```python
from build123d import *

# Parameters (mm, degrees)
F1_DEPTH = 0.75
F2_DEPTH = 1
F4_DEPTH = 0.75
F6_DEPTH = 0.75
F8_DEPTH = 0.75


with BuildPart() as f1:
    # F0 (on Top) → F1 (new body)
    with BuildSketch(Plane.XY):
        with BuildLine():
            add(Edge.make_bspline(
                [(-37.5, 18.7313321615), (-32.3807911431, 17.926577975), (-18.7011737223, 16.5680764405), (-7.3513992733, 15.9357535011), (0, 15.7313321615)],
                knots=[0, 0, 0, 0, 0.4901565124, 1, 1, 1, 1], degree=3))
            Line((-37.5, 18.7313321615), (-47, -23.1548529118))
            Line((-47, -23.1548529118), (-16.0084403101, -23.1548529118))
            Line((-16.0084403101, -23.1548529118), (-16.0063231241, -23.0646254072))
            add(Edge.make_bspline(
                [(-43.315390494, -20.4723017862), (-38.3905339247, -21.2993483436), (-33.0056838871, -22.2189238519), (-21.2861009313, -22.8925835376), (-16.0063231241, -23.0646254072)],
                knots=[0, 0, 0, 0, 0.398937465, 0.6969379575, 0.6969379575, 0.6969379575, 0.6969379575], degree=3))
            Line((-43.315390494, -20.4723017862), (-42.7131794367, -17.8171098074))
            Line((-42.7131794367, -17.8171098074), (-43.4446029246, -17.651219237))
            Line((-43.4446029246, -17.651219237), (-36.3666052528, 13.5561829132))
            Line((-36.3666052528, 13.5561829132), (-35.635181765, 13.3902923427))
            Line((-35.635181765, 13.3902923427), (-35.1425150574, 15.562495384))
            add(Edge.make_bspline(
                [(-35.1425150574, 15.562495384), (-30.4836686701, 14.6303577349), (-22.7091897663, 13.9291012054), (-15.9390947662, 13.4553124867), (-14.8013141006, 13.3810050341)],
                knots=[0, 0, 0, 0, 0.4908367268, 0.5909725979, 0.5909725979, 0.5909725979, 0.5909725979], degree=3))
            Line((-14.8013141006, 13.3810050341), (-14.8013141006, 14.1310050341))
            Line((-14.8013141006, 14.1310050341), (-8.8108518429, 13.792830613))
            Line((-8.8108518429, 13.792830613), (-8.8108518429, 13.042830613))
            add(Edge.make_bspline(
                [(-8.8108518429, 13.042830613), (-6.0913133604, 12.9141276056), (-3.2370188614, 12.8126642043), (0, 12.7313321615)],
                knots=[0.7661743328, 0.7661743328, 0.7661743328, 0.7661743328, 1, 1, 1, 1], degree=3))
            Line((0, 12.7313321615), (0, 15.7313321615))
        make_face()
        with BuildLine():
            Line((-16.0084403101, -23.1548529118), (-47, -23.1548529118))
            add(Edge.make_bspline(
                [(-47, -23.1548529118), (-39.471310208, -24.0545421828), (-29.2503257197, -25.7571688291), (-8.0323131497, -26.1634826516), (0, -26.1548529118)],
                knots=[0, 0, 0, 0, 0.4528935937, 1, 1, 1, 1], degree=3))
            Line((0, -26.1548529118), (0, -23.1548529118))
            add(Edge.make_bspline(
                [(-10.0079742572, -23.2053765011), (-6.5667353079, -23.2536816802), (-3.1521121944, -23.2431206783), (0, -23.1548529118)],
                knots=[0.8085428965, 0.8085428965, 0.8085428965, 0.8085428965, 1, 1, 1, 1], degree=3))
            Line((-10.0079742572, -23.2053765011), (-10.0255681439, -23.9551701095))
            Line((-10.0255681439, -23.9551701095), (-16.0239170108, -23.8144190156))
            Line((-16.0239170108, -23.8144190156), (-16.0084403101, -23.1548529118))
        make_face()
        with BuildLine():
            Line((-16.0063231241, -23.0646254072), (-16.0084403101, -23.1548529118))
            Line((-16.0084403101, -23.1548529118), (-12.748052928, -23.1548529118))
            add(Edge.make_bspline(
                [(-16.0063231241, -23.0646254072), (-14.9289009553, -23.0997332718), (-13.8402912127, -23.1300103495), (-12.748052928, -23.1548529118)],
                knots=[0.6969379575, 0.6969379575, 0.6969379575, 0.6969379575, 0.7577496714, 0.7577496714, 0.7577496714, 0.7577496714], degree=3))
        make_face()
        with BuildLine():
            Line((-12.748052928, -23.1548529118), (-16.0084403101, -23.1548529118))
            Line((-16.0084403101, -23.1548529118), (-16.0239170108, -23.8144190156))
            Line((-16.0239170108, -23.8144190156), (-10.0255681439, -23.9551701095))
            Line((-10.0255681439, -23.9551701095), (-10.0079742572, -23.2053765011))
            add(Edge.make_bspline(
                [(-12.748052928, -23.1548529118), (-11.8357565687, -23.1756027605), (-10.9209287599, -23.192561224), (-10.0079742572, -23.2053765011)],
                knots=[0.7577496714, 0.7577496714, 0.7577496714, 0.7577496714, 0.8085428965, 0.8085428965, 0.8085428965, 0.8085428965], degree=3))
        make_face()
        with BuildLine():
            add(Edge.make_bspline(
                [(-14.8013141006, 13.3810050341), (-12.8106074305, 13.2509937357), (-10.8485573953, 13.1392656642), (-8.8108518429, 13.042830613)],
                knots=[0.5909725979, 0.5909725979, 0.5909725979, 0.5909725979, 0.7661743328, 0.7661743328, 0.7661743328, 0.7661743328], degree=3))
            Line((-8.8108518429, 13.042830613), (-8.8108518429, 13.792830613))
            Line((-8.8108518429, 13.792830613), (-14.8013141006, 14.1310050341))
            Line((-14.8013141006, 14.1310050341), (-14.8013141006, 13.3810050341))
        make_face()
        Polygon((-43.4446029246, -17.651219237), (-42.7131794367, -17.8171098074), (-35.635181765, 13.3902923427), (-36.3666052528, 13.5561829132), align=None)
    extrude(amount=F1_DEPTH)

    # F0 (on Top) → F2 (join)
    with BuildSketch(Plane.XY):
        with BuildLine():
            Line((-16.0063231241, -23.0646254072), (-16.0084403101, -23.1548529118))
            Line((-16.0084403101, -23.1548529118), (-12.748052928, -23.1548529118))
            add(Edge.make_bspline(
                [(-16.0063231241, -23.0646254072), (-14.9289009553, -23.0997332718), (-13.8402912127, -23.1300103495), (-12.748052928, -23.1548529118)],
                knots=[0.6969379575, 0.6969379575, 0.6969379575, 0.6969379575, 0.7577496714, 0.7577496714, 0.7577496714, 0.7577496714], degree=3))
        make_face()
        with BuildLine():
            Line((-12.748052928, -23.1548529118), (-16.0084403101, -23.1548529118))
            Line((-16.0084403101, -23.1548529118), (-16.0239170108, -23.8144190156))
            Line((-16.0239170108, -23.8144190156), (-10.0255681439, -23.9551701095))
            Line((-10.0255681439, -23.9551701095), (-10.0079742572, -23.2053765011))
            add(Edge.make_bspline(
                [(-12.748052928, -23.1548529118), (-11.8357565687, -23.1756027605), (-10.9209287599, -23.192561224), (-10.0079742572, -23.2053765011)],
                knots=[0.7577496714, 0.7577496714, 0.7577496714, 0.7577496714, 0.8085428965, 0.8085428965, 0.8085428965, 0.8085428965], degree=3))
        make_face()
        with BuildLine():
            add(Edge.make_bspline(
                [(-14.8013141006, 13.3810050341), (-12.8106074305, 13.2509937357), (-10.8485573953, 13.1392656642), (-8.8108518429, 13.042830613)],
                knots=[0.5909725979, 0.5909725979, 0.5909725979, 0.5909725979, 0.7661743328, 0.7661743328, 0.7661743328, 0.7661743328], degree=3))
            Line((-8.8108518429, 13.042830613), (-8.8108518429, 13.792830613))
            Line((-8.8108518429, 13.792830613), (-14.8013141006, 14.1310050341))
            Line((-14.8013141006, 14.1310050341), (-14.8013141006, 13.3810050341))
        make_face()
        Polygon((-43.4446029246, -17.651219237), (-42.7131794367, -17.8171098074), (-35.635181765, 13.3902923427), (-36.3666052528, 13.5561829132), align=None)
    extrude(amount=-F2_DEPTH)

    # F3 (on face) → F4 (join, through all)
    with BuildSketch(Plane.XY.offset(0.75)):
        Polygon((-47.9752313172, -22.9336654846), (-47, -23.1548529118), (-37.5, 18.7313321615), (-38.4752313172, 18.9525195888), align=None)
    extrude(amount=-F4_DEPTH)

    # F5 (on face) → F6 (join, through all)
    with BuildSketch(Plane.XY.offset(0.75)):
        with BuildLine():
            Line((-38.1434501763, 20.4153665646), (-38.4752313172, 18.9525195888))
            Line((-38.4752313172, 18.9525195888), (-37.5, 18.7313321615))
            add(Edge.make_bspline(
                [(-37.5, 18.7313321615), (-32.3807911431, 17.926577975), (-18.7011737223, 16.5680764405), (-7.3513992733, 15.9357535011), (0, 15.7313321615)],
                knots=[0, 0, 0, 0, 0.4901565124, 1, 1, 1, 1], degree=3))
            Line((0, 15.7313321615), (0, 17.2313321615))
            Line((0, 17.2313321615), (-3.3217752352, 17.2313321615))
            Line((-3.3217752352, 17.2313321615), (-18.8273077893, 18.2105369309))
            Line((-18.8273077893, 18.2105369309), (-38.1434501763, 20.4153665646))
        make_face()
    extrude(amount=-F6_DEPTH)

    # F7 (on face) → F8 (join, through all)
    with BuildSketch(Plane.XY.offset(0.75)):
        with BuildLine():
            Line((-47, -23.1548529118), (-47.9752313172, -22.9336654846))
            Line((-47.9752313172, -22.9336654846), (-48.6002014355, -25.6892038047))
            Line((-48.6002014355, -25.6892038047), (-31.8084545434, -28.2887462527))
            Line((-31.8084545434, -28.2887462527), (-11.6026224568, -29.4112917036))
            Line((-11.6026224568, -29.4112917036), (0, -29.9293901771))
            Line((0, -29.9293901771), (0, -26.1548529118))
            add(Edge.make_bspline(
                [(-47, -23.1548529118), (-39.471310208, -24.0545421828), (-29.2503257197, -25.7571688291), (-8.0323131497, -26.1634826516), (0, -26.1548529118)],
                knots=[0, 0, 0, 0, 0.4528935937, 1, 1, 1, 1], degree=3))
        make_face()
    extrude(amount=-F8_DEPTH)

    # F9 (on face) → F11 section 0
    with BuildSketch(Plane.YZ.offset(-8.8108518429)):
        Polygon((13.792830613, -0.5), (13.792830613, -1), (15.6468802348, -1.75), (15.6468802348, -1.25), align=None)
    # F10 (on face) → F11 section 1
    with BuildSketch(Plane(origin=(-14.8013141006, 0, 0), x_dir=(0, -1, 0), z_dir=(-1, 0, 0))):
        Polygon((-15.9850546559, -1.75), (-14.1310050341, -1), (-14.1310050341, -0.5), (-15.9850546559, -1.25), align=None)
    loft()

    # F12 (on face) → F14 section 0
    with BuildSketch(Plane(origin=(-15.4566018313, 0.3626887438, 0), x_dir=(-0.0234585156, -0.9997248112, 0), z_dir=(-0.9997248112, 0.0234585156, 0))):
        Polygon((24.1837628611, -0.5), (24.1837628611, -1), (26.0378124829, -1.75), (26.0378124829, -1.25), align=None)
    # F13 (on face) → F14 section 1
    with BuildSketch(Plane(origin=(-9.4582529644, 0.2219376499, 0), x_dir=(0.0234585156, 0.9997248112, 0), z_dir=(0.9997248112, -0.0234585156, 0))):
        Polygon((-26.0378124829, -1.75), (-24.1837628611, -1), (-24.1837628611, -0.5), (-26.0378124829, -1.25), align=None)
    loft()

    # F15 (on face) → F17 section 0
    with BuildSketch(Plane(origin=(1.1449940284, 5.04836124, 0), x_dir=(-0.9752313172, 0.2211874272, 0), z_dir=(0.2211874272, 0.9752313172, 0))):
        Polygon((38.4643095643, -0.5), (38.4643095643, -1), (40.3183591861, -1.75), (40.3183591861, -1.25), align=None)
    # F16 (on face) → F17 section 1
    with BuildSketch(Plane(origin=(-5.9330036433, -26.1590409101, 0), x_dir=(0.9752313172, -0.2211874272, 0), z_dir=(-0.2211874272, -0.9752313172, 0))):
        Polygon((-40.3183591861, -1.75), (-38.4643095643, -1), (-38.4643095643, -0.5), (-40.3183591861, -1.25), align=None)
    loft()

    # F18: F1 across plane


with BuildPart() as f1_1:
    add(f1.part)
    add(f1.part.mirror(Plane.YZ))


solid = f1_1.part
```
Check sheet for the modelled part. Datum: model origin and axes. Units: mm. A direction names the side the tool comes from. Give positions to 0.01 mm unless a question says otherwise; leave off trailing zeros. Return JSON: item names as keys, results as strings.
1. Mould release check, pull along X, two halves, no side actions. Record for faces 5 (the flat face through (28.35, 19.298, 0.38)), 6 (the flat face through (43.609, -17.614, -0.856)), 7 (the flat face through (-3, -25, 0.75)), 8 (the flat face through (-40.32, -26.97, 0.38)): +X half, -X half, draft (parallel to the pull), parting line (faces both ways), or undercut.
From the geometry:
{"face 5": "undercut", "face 6": "+X half", "face 7": "draft", "face 8": "-X half"}
2. Material ranges on probe 1 along X at (y, z) = (-16.5, -0.2); probe 2 along X at (y, z) = (-12, 0.65); probe 3 along Y at (x, z) = (4, 0.2), recorded low to high. Write a range as [from, to].
From the geometry:
{"probe 1": "[-43.18, -42.41], [42.41, 43.18]", "probe 2": "[-45.5, -41.39], [41.39, 45.5]", "probe 3": "[-29.75, -23.23], [12.85, 17.27]"}
3. Set-up check for faces 1 (the flat face through (-43.609, -17.614, -0.856)), 2 (the flat face through (-39.856, -1.829, -0.246)), 3 (the flat face through (39.6, -2.1, -1)), 4 (the flat face through (39.856, -1.829, -0.246)): record each of +Z, -Z, +X, -X, +Y, -Y from which the full face is reachable in a straight line by a thin tool's end or side.
From the geometry:
{"face 1": "-Z, -X, -Y", "face 2": "-X, +Y", "face 3": "-Z, -Y", "face 4": "+X, +Y"}
4. Go/stop test with flat-tipped pins: P1, Ø6, axis at x = -39, y = -5, coming from the -Z side; P2, Ø4, axis at x = 38, y = 5, coming from the -Z side; P3, Ø1.2, axis at x = -11, y = 13.5, coming from the -Z side. Record where each tip stops, or that it passes through.
From the geometry:
{"P1": "z = -1.59", "P2": "z = -1.69", "P3": "z = -1.07"}
